Geometry: final body of the model. Coordinates: model frame, mm. A direction names the side the tool comes from. Coordinates: 2 decimals unless noted, no trailing zeros. Loops run counter-clockwise (first coordinate to the right, second up) from the corner with the lowest first, then second, coordinate; pieces in that order, holes last. Notation, with made-up numbers: (-2, 86) - (52, 86) arc R7 cw to (52, 92) - close; hole circle Ø4 at (44.25, 47.25). An arc over 180 degrees is marked (long way). Answer in a Markdown table with one row per item.
from build123d import *

# Parameters (mm, degrees)
F1_DEPTH = 3


with BuildPart() as f1:
    # F0 (on Front) → F1 (new body)
    with BuildSketch(Plane.XZ):
        with BuildLine():
            Line((13, 15), (13, 30))
            ThreePointArc((13, 30), (0, 43), (-13, 30))
            Line((-13, 30), (-13, 15))
            Line((-13, 15), (-10, 15))
            Line((-10, 15), (-10, 7))
            Line((-10, 7), (-13, 7))
            Line((-13, 7), (-13, 0))
            Line((-13, 0), (-9, 0))
            Line((-9, 0), (-9, -3))
            Line((-9, -3), (-2, -3))
            Line((-2, -3), (-2, 0))
            Line((-2, 0), (0, 0))
            Line((0, 0), (2, 0))
            Line((2, 0), (2, -3))
            Line((2, -3), (9, -3))
            Line((9, -3), (9, 0))
            Line((9, 0), (13, 0))
            Line((13, 0), (13, 7))
            Line((13, 7), (10, 7))
            Line((10, 7), (10, 15))
            Line((10, 15), (13, 15))
        make_face()
        with BuildLine():
            ThreePointArc((-7.549834, 22), (-11, 30), (-7.549834, 38))
            Line((-7.549834, 38), (7.549834, 38))
            ThreePointArc((7.549834, 38), (11, 30), (7.549834, 22))
            Line((7.549834, 22), (-7.549834, 22))
        make_face(mode=Mode.SUBTRACT)
    extrude(amount=F1_DEPTH)


solid = f1.part
(1) Cut plane B-B on y = -1.4. Output: boundary loops of the cut face in (x, z), then the cut area to 3 significant figures.
Verdict:
| item | result |
|---|---|
| outline | (-13, 0) - (-9, 0) - (-9, -3) - (-2, -3) - (-2, 0) - (2, 0) - (2, -3) - (9, -3) - (9, 0) - (13, 0) - (13, 7) - (10, 7) - (10, 15) - (13, 15) - (13, 30) arc R13 ccw to (-13, 30) - (-13, 15) - (-10, 15) - (-10, 7) - (-13, 7) - close; hole (-7.55, 22) - (7.55, 22) arc R11 ccw to (7.55, 38) - (-7.55, 38) arc R11 ccw to start |
| area | 722 mm² |
(2) Cut plane A-A on x = 1.5. Output: boundary loops of the cut face in (y, z), then the cut area to 3 significant figures.
Verdict:
| item | result |
|---|---|
| outline | (-3, 0) - (0, 0) - (0, 22) - (-3, 22) - close; (-3, 38) - (0, 38) - (0, 42.91) - (-3, 42.91) - close |
| area | 80.7 mm² |
(3) Access query for faces 4 (the face through (2, -1, -1)), 5 (the face through (-11, -1, 7)), 6 (the face through (0, -1, 38)), 7 (the face through (10, -1, 11)), 8 (the face through (9, -1, -2)). Directions: +Z, -Z, +X, -X, +Y, -Y. A direction counts if a zero-diameter tool reaches every point of the face in a straight line with its end or side. Return the directions, or none.
Verdict:
| item | result |
|---|---|
| face 4 | -Z, +Y, -Y |
| face 5 | -X, +Y, -Y |
| face 6 | +Y, -Y |
| face 7 | +X, +Y, -Y |
| face 8 | -Z, +X, +Y, -Y |
(4) Ray query, probe 1 along X at (y, z) = (-1.9, 30); probe 2 along Z at (x, y) = (0.5, -2.1); probe 3 along Z at (x, y) = (6, -1.65). Return the intervals inside material, ascending.
Verdict:
| item | result |
|---|---|
| probe 1 | x = -13 to -11, 11 to 13 |
| probe 2 | z = 0 to 22, 38 to 42.99 |
| probe 3 | z = -3 to 22, 38 to 41.53 |
(5) Cut plane C-C on z = 33.5. Output: boundary loops of the cut face in (x, y).
Verdict:
| item | result |
|---|---|
| outline | (-12.52, -3) - (-10.43, -3) - (-10.43, 0) - (-12.52, 0) - close; (10.43, -3) - (12.52, -3) - (12.52, 0) - (10.43, 0) - close |
(6) Pull-direction query (Z, two-part tool) for faces 1 (the face through (0, -1, 43)), 2 (the face through (-13, -1, 4)), 3 (the face through (-10, -1, 11)); classes: pulls with the +Z half, pulls with the -Z half, needs draft (parallel to the pull), parting line crosses it, or undercut.
Verdict:
| item | result |
|---|---|
| face 1 | pulls with the +Z half |
| face 2 | needs draft |
| face 3 | undercut |
(7) First-contact query: pin 1 Ø0.9 at (y, z) = (-1, -1) entering from +X; pin 2 Ø0.9 at (x, y) = (-3.5, -2) entering from +Z; pin 3 Ø1.5 at (x, y) = (-10.5, -2) entering from -Z. Flat tips, straight axial feed; report the tip coordinate or a pass-through.
Verdict:
| item | result |
|---|---|
| pin 1 | stops at x = 9 |
| pin 2 | stops at z = 42.64 |
| pin 3 | stops at z = 0 |
